from build123d import *

# Parameters (mm, degrees)
VOLUME_KNOB_R                      = 35
KNOB_TOP_DEPTH                     = 3.5
VOLUME_KNOB_3_R                    = 35
VOLUME_KNOB_3_R_2                  = 32
KNOB_WALLS_DEPTH                   = 26
KNOB_START                         = 3.5
KNOB_SHAFT_KEYWAY_DEPTH            = 10
VOLUME_KNOB_8_R                    = 29.33
VOLUME_KNOB_8_R_2                  = 3
KNOB_DAMEPNING_EXTENSION_TOP_DEPTH = 12.9
KNOB_START_2                       = 16.4
VOLUME_KNOB_11_R                   = 10
VOLUME_KNOB_11_R_2                 = 3
KNOB_SHAFT_SUPPORT_DEPTH           = 5
SKETCH1_R                          = 5.75
WEIGHT_SLUG_HOLES_DEPTH            = 12.7


with BuildPart() as part:
    # Volume Knob → Knob Top (new body)
    with BuildSketch(Plane(origin=(0, 0, 0), x_dir=(1, 0, 0), z_dir=(0, 1, 0))):
        with Locations(Location((0, 0, 0), (0, 0, 270))):
            Circle(VOLUME_KNOB_R)
    extrude(amount=KNOB_TOP_DEPTH)

    # Volume Knob<3> → Knob Walls (add)
    with BuildSketch(Plane(origin=(0, 0, 0), x_dir=(1, 0, 0), z_dir=(0, 1, 0))):
        with Locations(Location((0, 0, 0), (0, 0, 270))):
            Circle(VOLUME_KNOB_3_R)
        with Locations(Location((0, 0, 0), (0, 0, 90))):
            Circle(VOLUME_KNOB_3_R_2, mode=Mode.SUBTRACT)
    extrude(amount=KNOB_WALLS_DEPTH)

    # Volume Knob<4> → Knob Shaft Keyway (add)
    with BuildSketch(Plane(origin=(0, 0, 0), x_dir=(1, 0, 0), z_dir=(0, 1, 0)).offset(KNOB_START)):
        with BuildLine():
            Line((-2.598076211, 1.5), (2.598076211, 1.5))
            ThreePointArc((2.598076211, 1.5), (0, 3), (-2.598076211, 1.5))
        make_face()
    extrude(amount=KNOB_SHAFT_KEYWAY_DEPTH)

    # Volume Knob<8> → Knob Damepning Extension (top) (add)
    with BuildSketch(Plane(origin=(0, 0, 0), x_dir=(1, 0, 0), z_dir=(0, 1, 0)).offset(KNOB_START)):
        with Locations(Location((0, 0, 0), (0, 0, 90))):
            Circle(VOLUME_KNOB_8_R)
        with Locations(Location((0, 0, 0), (0, 0, 150))):
            Circle(VOLUME_KNOB_8_R_2, mode=Mode.SUBTRACT)
    extrude(amount=KNOB_DAMEPNING_EXTENSION_TOP_DEPTH)

    # Volume Knob<11> → Knob Shaft Support (add)
    with BuildSketch(Plane(origin=(0, 0, 0), x_dir=(1, 0, 0), z_dir=(0, 1, 0)).offset(KNOB_START_2)):
        with Locations(Location((0, 0, 0), (0, 0, 270))):
            Circle(VOLUME_KNOB_11_R)
        with Locations(Location((0, 0, 0), (0, 0, 150))):
            Circle(VOLUME_KNOB_11_R_2, mode=Mode.SUBTRACT)
    extrude(amount=KNOB_SHAFT_SUPPORT_DEPTH)

    # Sketch1 → Weight Slug Holes (cut)
    with BuildSketch(Plane(origin=(0, 16.4, 0), x_dir=(1, 0, 0), z_dir=(0, 1, 0))):
        with Locations(Location((19.665, 0, 0), (0, 0, 270))):
            Circle(SKETCH1_R)
        with Locations(Location((12.260926954, -15.374716103, 0), (0, 0, 270))):
            Circle(SKETCH1_R)
        with Locations(Location((-4.375874166, -19.171957393, 0), (0, 0, 270))):
            Circle(SKETCH1_R)
        with Locations(Location((-17.717552787, -8.53232373, 0), (0, 0, 270))):
            Circle(SKETCH1_R)
        with Locations(Location((-17.717552787, 8.53232373, 0), (0, 0, 270))):
            Circle(SKETCH1_R)
        with Locations(Location((-4.375874166, 19.171957393, 0), (0, 0, 270))):
            Circle(SKETCH1_R)
        with Locations(Location((12.260926954, 15.374716103, 0), (0, 0, 270))):
            Circle(SKETCH1_R)
    extrude(amount=-WEIGHT_SLUG_HOLES_DEPTH, mode=Mode.SUBTRACT)


solid = part.part
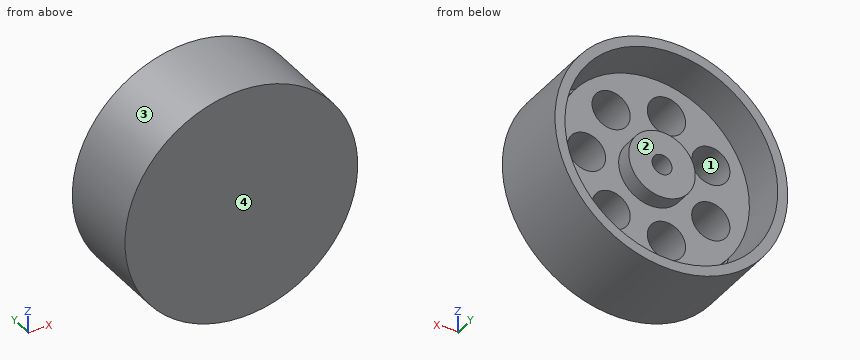
Can you work these out from the model? Positions are in its coordinate system, mm. Face numbers are marked on the shaded views. Round coordinates to 2 decimals unless told otherwise and drop trailing zeros. Write each loop counter-clockwise with the first axis right and the second up, starting at its lowest first coordinate (ties: lowest second). Pieces come first, ordered by that corner, then holes. Notation, with made-up numbers: (13.25, 63) -> (46.25, 63) arc R26 cw to (46.25, 87) -> close; hole circle Ø2 at (87.5, -20.5). An arc over 180 degrees is marked (long way). Use one line per item in the form item = value. Start each with the question number.
Q1. Imagine slicing it at B-B (z = 28). Please give me the cut outline in (x, y).
Q2. If I drill on probe 1 along X at (y, z) = (16.5, 0); probe 2 along X at (y, z) = (7, 0) (3 decimals); probe 3 along X at (y, z) = (15, 1.5), over which ranges is the centre line in solid material (lowest first)? Write a range as [from, to].
Q3. Imagine slicing it at A-A (y = 5.25). Count the separate pieces of the cut face and the enclosed holes in it, then the cut area to 3 significant figures.
Q4. We'd pull the mould along X, two halves only. Please class the marked faces 1, 2, 3 and 4: +X half, -X half, draft (parallel to the pull), parting line (faces both ways), or undercut.
Q5. I'm going to push flat-ended pins straight in: P1, Ø9, axis at x = 19.665, z = 0, coming from the +Y side; P2, Ø0.8, axis at x = -0.5, z = -2, coming from the +Y side; P3, Ø5, axis at x = 3.5, z = 6.5, coming from the +Y side. Where does each tip first touch, or does it pass through?
Q6. Imagine slicing it at C-C (x = 11). Please give me the cut outline in (y, z), then the cut area to 3 significant figures.
Q7. Imagine slicing it at D-D (z = 0). Please give me the cut outline in (x, y) (3 decimals), then the cut area to 3 significant figures.
Worked out:
q1.outline = (-21, 0) -> (21, 0) -> (21, 26) -> (15.49, 26) -> (15.49, 3.5) -> (8.73, 3.5) -> (8.73, 16.4) -> (-8.73, 16.4) -> (-8.73, 3.5) -> (-15.49, 3.5) -> (-15.49, 26) -> (-21, 26) -> close
q2.probe_1 = [-35, -32], [-10, -3], [3, 10], [32, 35]
q2.probe_2 = [-35, -32], [-29.33, -3], [3, 13.915], [25.415, 29.33], [32, 35]
q2.probe_3 = [-34.97, -31.96], [-29.29, -2.6], [2.6, 14.11], [25.22, 29.29], [31.96, 34.97]
q3.separate_pieces = 2
q3.enclosed_holes = 9
q3.area = 2,580 mm^2
q4.face_1 = undercut
q4.face_2 = undercut
q4.face_3 = parting line
q4.face_4 = draft
q5.P1 = 3.7
q5.P2 = 13.5
q5.P3 = 21.4
q6.outline = (0, -33.23) -> (26, -33.23) -> (26, -30.05) -> (3.5, -30.05) -> (3.5, -27.19) -> (16.4, -27.19) -> (16.4, -20.98) -> (3.7, -20.98) -> (3.7, -9.76) -> (16.4, -9.76) -> (16.4, 9.76) -> (3.7, 9.76) -> (3.7, 20.98) -> (16.4, 20.98) -> (16.4, 27.19) -> (3.5, 27.19) -> (3.5, 30.05) -> (26, 30.05) -> (26, 33.23) -> (0, 33.23) -> close
q6.area = 792 mm^2
q7.outline = (-35, 0) -> (35, 0) -> (35, 26) -> (32, 26) -> (32, 3.5) -> (29.33, 3.5) -> (29.33, 16.4) -> (25.415, 16.4) -> (25.415, 3.7) -> (13.915, 3.7) -> (13.915, 16.4) -> (10, 16.4) -> (10, 21.4) -> (3, 21.4) -> (3, 3.5) -> (-3, 3.5) -> (-3, 21.4) -> (-10, 21.4) -> (-10, 16.4) -> (-29.33, 16.4) -> (-29.33, 3.5) -> (-32, 3.5) -> (-32, 26) -> (-35, 26) -> close
q7.area = 983 mm^2
